For this review, use the dimensioned drawing (mm, ordinates from the lowest corner) and the shaded views. A direction names the side the tool comes from. Round coordinates to 2 decimals unless told otherwise and drop trailing zeros. Order: outer loops, then holes, each group sorted by start corner. A loop starts at its lowest first (then second) coordinate and runs counter-clockwise, first axis right, second up. Notation, with made-up numbers: (25, 11.5) - (67, 11.5) arc R20 cw to (67, 42.5) - close; hole circle Ø11 at (9.25, 65). An arc over 180 degrees is marked (long way). Write each question's results on one line, items separated by ' | '. Start each with the question number.
(1) For L1, parallel to Y at x = 2.35, z = 60; L2, parallel to X at y = 10, z = 56.5; L3, parallel to Z at x = 69, y = 25.5, list the stretches that pass through material, from the lowest coordinate up. Write a range as from..to.
(2) Take a section at B-B, the plane y = 12. Give the boundary of the cut face in (x, z), plus the area to 3 significant figures.
(3) For the marked faces 1, 2 and 3, list the 3-axis set-ups (+Z, -Z, +X, -X, +Y, -Y) from which the entire face can be reached by the end or side of a thin tool; tool diameter is ignored.
(4) Take a section at A-A, the plane z = 60. Give the boundary of the cut face in (x, y).
(5) Take a section at C-C, the plane x = 11.5. Give the boundary of the cut face in (y, z), plus the area to 3 significant figures.
(6) Insertion check: pin 1 Ø16.5 at (x, y) = (54.5, 23.5) entering from -Z; pin 2 Ø12 at (x, z) = (65, 44.5) entering from +Y; pin 3 Ø3 at (x, z) = (26.5, 22) entering from -Y. Each pin has a flat end and moves straight along its axis. Give the tip position at first contact, or say it passes through.
(7) Take a section at D-D, the plane z = 44. Give the boundary of the cut face in (x, y).
(8) Draft analysis for pull direction X (two halves, no side actions). For the marked faces 4, 5, 6 and 7, state which applies: pulls with the +X half, pulls with the -X half, needs draft (parallel to the pull), parting line crosses it, or undercut.
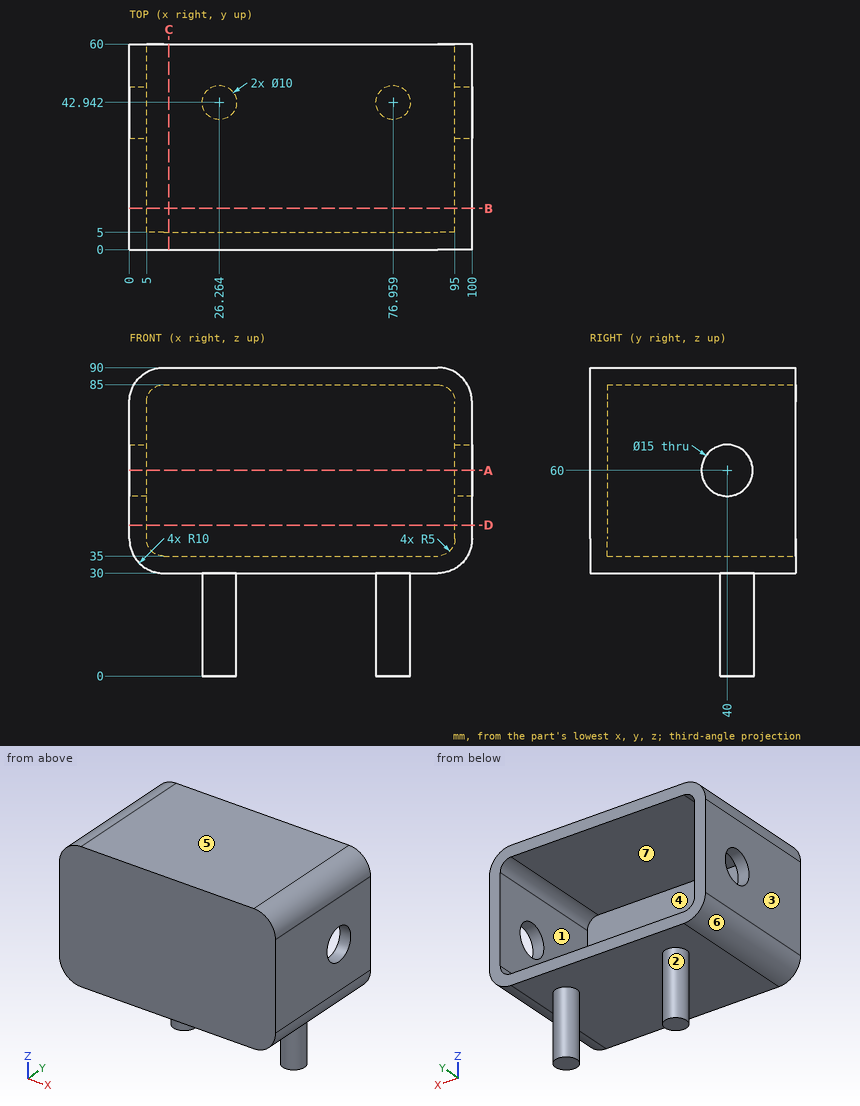
Results below:
1) L1: y = 0..32.5, 47.5..60 | L2: x = 0..5, 95..100 | L3: z = 30..35, 85..90
2) outline: (0, 40) arc R10 ccw to (10, 30) - (90, 30) arc R10 ccw to (100, 40) - (100, 80) arc R10 ccw to (90, 90) - (10, 90) arc R10 ccw to (0, 80) - close; hole (5, 40) arc R5 ccw to (10, 35) - (90, 35) arc R5 ccw to (95, 40) - (95, 80) arc R5 ccw to (90, 85) - (10, 85) arc R5 ccw to (5, 80) - close | area: 1,440 mm^2
3) face 1: +Y | face 2: -Z | face 3: +Z, -Z, -X, +Y, -Y
4) outline: (0, 0) - (100, 0) - (100, 32.5) - (95, 32.5) - (95, 5) - (5, 5) - (5, 32.5) - (0, 32.5) - close; (0, 47.5) - (5, 47.5) - (5, 60) - (0, 60) - close; (95, 47.5) - (100, 47.5) - (100, 60) - (95, 60) - close
5) outline: (0, 30) - (60, 30) - (60, 35) - (5, 35) - (5, 85) - (60, 85) - (60, 90) - (0, 90) - close | area: 850 mm^2
6) pin 1: stops at z = 30 | pin 2: stops at y = 5 | pin 3: stops at y = 37.94
7) outline: (0, 0) - (100, 0) - (100, 60) - (95, 60) - (95, 5) - (5, 5) - (5, 60) - (0, 60) - close
8) face 4: undercut | face 5: needs draft | face 6: pulls with the -X half | face 7: undercut
